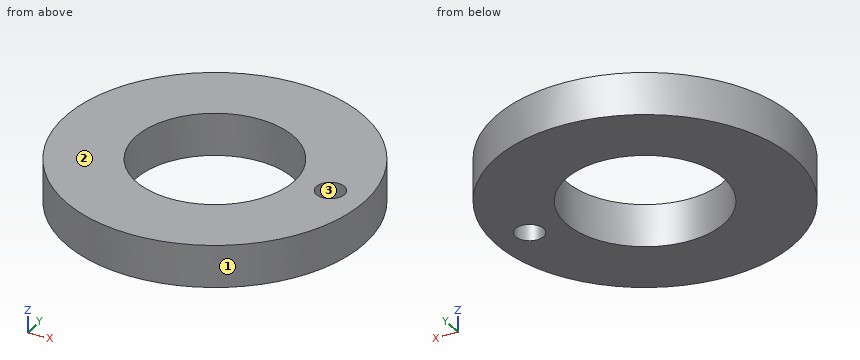
from build123d import *

# Parameters (mm, degrees)
CYLINDER_R      = 10.6
CYLINDER_DEPTH  = 3
SKETCH_R        = 5.6
POCKET_DEPTH    = 3
SKETCH001_R     = 1
POCKET001_DEPTH = 3


with BuildPart() as part:
    # Cylinder → Cylinder (new body)
    with BuildSketch(Plane.XY):
        Circle(CYLINDER_R)
    extrude(amount=CYLINDER_DEPTH)

    # Sketch → Pocket (cut)
    with BuildSketch(Plane.XY.offset(3)):
        Circle(SKETCH_R)
    extrude(amount=-POCKET_DEPTH, mode=Mode.SUBTRACT)

    # Sketch001 → Pocket001 (cut)
    with BuildSketch(Plane.XY.offset(3)):
        with Locations((8.1, 0)):
            Circle(SKETCH001_R)
    extrude(amount=-POCKET001_DEPTH, mode=Mode.SUBTRACT)


solid = part.part
The model under review builds one solid part; all positions refer to its coordinate system, in mm. Face numbers are marked on the shaded views. Round coordinates to 2 decimals unless told otherwise and drop trailing zeros. Write each loop counter-clockwise with the first axis right and the second up, starting at its lowest first coordinate (ties: lowest second). Pieces come first, ordered by that corner, then holes. Notation, with made-up numbers: M 84,41.25 L 131,41.25 A29 cw 131,71.25 Z; hole C -35,-15 d5. An arc over 180 degrees is marked long. Use a Markdown table: item, result. Add a question column.
Q1. The part is to be moulded in two halves that separate along Y. For the marked faces 1, 2 and 3, say which applies: pulls with the +Y half, pulls with the -Y half, needs draft (parallel to the pull), parting line crosses it, or undercut.
Q2. To check wall thickness, follow line 1 (X direction, y = -0.5, z = 1.05); line 2 (Y direction, x = 0, z = 1.75); line 3 (Y direction, x = 3, z = 1.9). State the ranges of each line that lie inside material, in increasing order.
Q3. We need section D-D, the plane y = 5. State the section outline as (x, z) points, plus the area to 3 significant figures.
Q4. We need section A-A, the plane x = 0. State the section outline as (y, z) points.
Q5. We need section C-C, the plane z = 0.85. State the section outline as (x, y) points, plus the area to 3 significant figures.
Q6. We need section B-B, the plane y = 0. State the section outline as (x, z) points.
Findings below:
| question | item | result |
|---|---|---|
| 1 | face 1 | parting line crosses it |
| 1 | face 2 | needs draft |
| 1 | face 3 | undercut |
| 2 | line 1 | x = -10.59 to -5.58, 5.58 to 7.23, 8.97 to 10.59 |
| 2 | line 2 | y = -10.6 to -5.6, 5.6 to 10.6 |
| 2 | line 3 | y = -10.17 to -4.73, 4.73 to 10.17 |
| 3 | outline | M -9.35,0 L -2.52,0 L -2.52,3 L -9.35,3 Z; M 2.52,0 L 9.35,0 L 9.35,3 L 2.52,3 Z |
| 3 | area | 40.9 mm² |
| 4 | outline | M -10.6,0 L -5.6,0 L -5.6,3 L -10.6,3 Z; M 5.6,0 L 10.6,0 L 10.6,3 L 5.6,3 Z |
| 5 | outline | C 0,0 d21.2; hole C 0,0 d11.2; hole C 8.1,0 d2 |
| 5 | area | 251 mm² |
| 6 | outline | M -10.6,0 L -5.6,0 L -5.6,3 L -10.6,3 Z; M 5.6,0 L 7.1,0 L 7.1,3 L 5.6,3 Z; M 9.1,0 L 10.6,0 L 10.6,3 L 9.1,3 Z |
